Autodesk Inventor part; units mm, degrees
ref_plane "YZ Plane" through (0, 0, 0) normal (1, 0, 0) x (0, 1, 0)
ref_plane "XZ Plane" through (0, 0, 0) normal (0, 1, 0) x (-1, 0, 0)
ref_plane "XY Plane" through (0, 0, 0) normal (0, 0, 1) x (1, 0, 0)
sketch "Sketch1" plane through (0, 0, 0) normal (0, 1, 0) x (-1, 0, 0)
  circle A0 centre (-15.2763, 11.7192) radius 2.1844
  circle A1 centre (46.1983, -4.1823) radius 2.1844
  circle A2 centre (-0.2854, 25.8488) radius 2.1844
  circle A3 centre (17.6488, 27.2646) radius 2.1844
  circle A4 centre (23.5893, -10.3689) radius 2.1844
  circle A5 centre (-38.3261, 27.9733) radius 2.1844
  circle A6 centre (-38.3261, 27.9733) radius 6.35
  circle A7 centre (23.5893, -10.3689) radius 6.35
  line L0 (-41.6694, 22.5746) -> (20.246, -15.7676)
  circle A8 centre (46.1983, -4.1823) radius 6.35
  line L1 (17.6488, 27.2646) -> (30.1935, 29.2448)
  circle A9 centre (36.1339, -8.3887) radius 6.35
  line L2 (48.647, -10.0412) -> (38.5826, -14.2476)
  line L3 (36.1339, -14.7387) -> (24.621, -16.6345)
  circle A10 centre (30.1935, 29.2448) radius 6.35
  line L4 (51.9256, -1.4401) -> (35.9208, 31.987)
  line L5 (-38.444, 34.3222) -> (30.0757, 35.5937)
  point P0 (0, 0)
  point P1 (17.7292, 33.6141)
  point P2 (-38.2458, 34.3228)
  point P3 (21.7554, 32.108)
  point P4 (24.1332, -16.6956)
  point P5 (50.8998, 0.086)
  point P6 (22.3503, 31.5329)
  point P7 (47.8742, -10.3072)
  point P8 (25.2652, -16.4937)
  dimension "d0" = 12.7
  dimension "d1" = 12.7
  dimension "d10" = 12.7
  dimension "d11" = 12.7
  dimension "d12" = 12.7
  dimension "d13" = 12.7
extrude "Extrusion1" add sketch "Sketch1" along normal blind 1.5875
properties part number "newsidepolytest2"
Here's how the part is built. I have some questions about the finished solid (model axes, mm). Round coordinates to 2 decimals unless told otherwise and drop trailing zeros. Loops run counter-clockwise (first coordinate to the right, second up) from the corner with the lowest first, then second, coordinate; pieces in that order, holes last.
1. For P1, Ø3, axis at x = 9, z = 11, coming from the -Y side; P2, Ø4, axis at x = 0.29, z = 25.85, coming from the +Y side, each with a flat end and sliding along its axis, tell me the tip position at first contact or that it passes through.
Answer list:
P1: stops at y = 0
P2: passes through
2. If I drill on line 1 along X through (y, z) = (1.25, 27); line 2 along X through (y, z) = (1.1, 25.5); line 3 along Z through (x, y) = (-30, 0.6), over which ranges is the centre line in solid material (lowest first)?
Answer list:
line 1: x = -38.31 to -19.82, -15.48 to -1.57, 2.14 to 36.37, 40.28 to 44.6
line 2: x = -39.03 to -18.94, -16.36 to -1.87, 2.44 to 44.17
line 3: z = -15.75 to 35.59
3. If we section it at B-B on z = 7: Write out the boundary of the cut face in (x, y).
Answer list:
outline: (-47.88, 0) - (16.52, 0) - (16.52, 1.59) - (-47.88, 1.59) - close
4. We'd pull the mould along Z, two halves only. Please class faces 1 (the face through (-14, 0, 16)), 2 (the face through (-30.458, 0.783, -15.673)), 3 (the face through (-44.465, 0.783, -2.853)): +Z half, -Z half, draft (parallel to the pull), parting line (faces both ways), or undercut.
Answer list:
face 1: draft
face 2: -Z half
face 3: undercut
5. If we section it at C-C on x = -31: Write out the boundary of the cut face in (y, z).
Answer list:
outline: (0, -15.58) - (1.59, -15.58) - (1.59, 35.54) - (0, 35.54) - close
6. If we section it at A-A on y = 1.05: Write out the boundary of the cut face in (x, z).
Answer list:
outline: (-51.93, -1.44) arc R6.35 ccw to (-48.65, -10.04) - (-38.58, -14.25) arc R6.35 ccw to (-36.13, -14.74) - (-24.62, -16.63) arc R6.35 ccw to (-20.25, -15.77) - (41.67, 22.57) arc R6.35 ccw to (38.44, 34.32) - (-30.08, 35.59) arc R6.35 ccw to (-35.92, 31.99) - close; hole circle Ø4.37 at (-46.2, -4.18); hole circle Ø4.37 at (-23.59, -10.37); hole circle Ø4.37 at (-17.65, 27.26); hole circle Ø4.37 at (0.29, 25.85); hole circle Ø4.37 at (15.28, 11.72); hole circle Ø4.37 at (38.33, 27.97)
